Can you work these out from the model? Positions are in its coordinate system, mm. Give positions to 0.01 mm unless a question says otherwise; leave off trailing zeros. Order: outer loops, then holes, each group sorted by start corner. A loop starts at its lowest first (then second) coordinate and runs counter-clockwise, first axis right, second up. Notation, with made-up numbers: (55.5, -26) -> (103.5, -26) arc R15 cw to (103.5, -7) -> close; hole circle Ø1 at (76, 61). An arc over 180 degrees is marked (long way). Answer as CSV lines item,"result".
```python
from build123d import *

# Parameters (mm, degrees)
F1_DEPTH = 38.1
F3_D     = 34.12998


with BuildPart() as f1:
    # F0 (on Top) → F1 (new body)
    with BuildSketch(Plane.XY):
        with BuildLine():
            ThreePointArc((119.0625, -25.4), (144.4625, 0), (119.0625, 25.4))
            Line((119.0625, 25.4), (-119.0625, 25.4))
            Line((-119.0625, 25.4), (-119.0625, -25.4))
            Line((-119.0625, -25.4), (119.0625, -25.4))
        make_face()
    extrude(amount=F1_DEPTH)

    # F3 (through all)
    with Locations(Plane.XY.offset(38.1)):
        with Locations((119.0625, 0)):
            Hole(F3_D / 2)


solid = f1.part
```
Item 1: Imagine slicing it at C-C, the plane x = 107.5. Please give me the cut outline in (y, z), then the cut area to 3 significant figures.
Numbers:
outline,"(-25.4, 0) -> (-12.55, 0) -> (-12.55, 38.1) -> (-25.4, 38.1) -> close; (12.55, 0) -> (25.4, 0) -> (25.4, 38.1) -> (12.55, 38.1) -> close"
area,"979 mm²"
Item 2: Please list where these lines run through material, in increasing order: line 1 along X through (y, z) = (15, 26); line 2 along X through (y, z) = (12.5, 26).
Numbers:
line 1,"x = -119.06 to 110.93, 127.2 to 139.56"
line 2,"x = -119.06 to 107.45, 130.68 to 141.17"
Item 3: For pin 1 (10 mm diameter, centred on y = 11.5, z = 9.5, fed in from +X), with a flat end and sliding along its axis, tell me the tip position at first contact or that it passes through.
Numbers:
pin 1,"stops at x = 143.62"
Item 4: Imagine slicing it at B-B, the plane z = 15. Please give me the cut outline in (x, y) (1 decimal).
Numbers:
outline,"(-119.1, -25.4) -> (119.1, -25.4) arc R25.4 ccw to (119.1, 25.4) -> (-119.1, 25.4) -> close; hole circle Ø34.1 at (119.1, 0)"
Item 5: We'd pull the mould along Y, two halves only. Please class faces 1 (the flat face through (11, 0, 38.1)), 2 (the flat face through (2, 25.4, 19)), 3 (the cylindrical face through (102.786, 5.126, 18.783)): released by +Y, released by -Y, zero draft, split by the parting line, or undercut.
Numbers:
face 1,"zero draft"
face 2,"released by +Y"
face 3,"undercut"
Item 6: Imagine slicing it at A-A, the plane y = 0. Please give me the cut outline in (x, z).
Numbers:
outline,"(-119.06, 0) -> (102, 0) -> (102, 38.1) -> (-119.06, 38.1) -> close; (136.13, 0) -> (144.46, 0) -> (144.46, 38.1) -> (136.13, 38.1) -> close"
